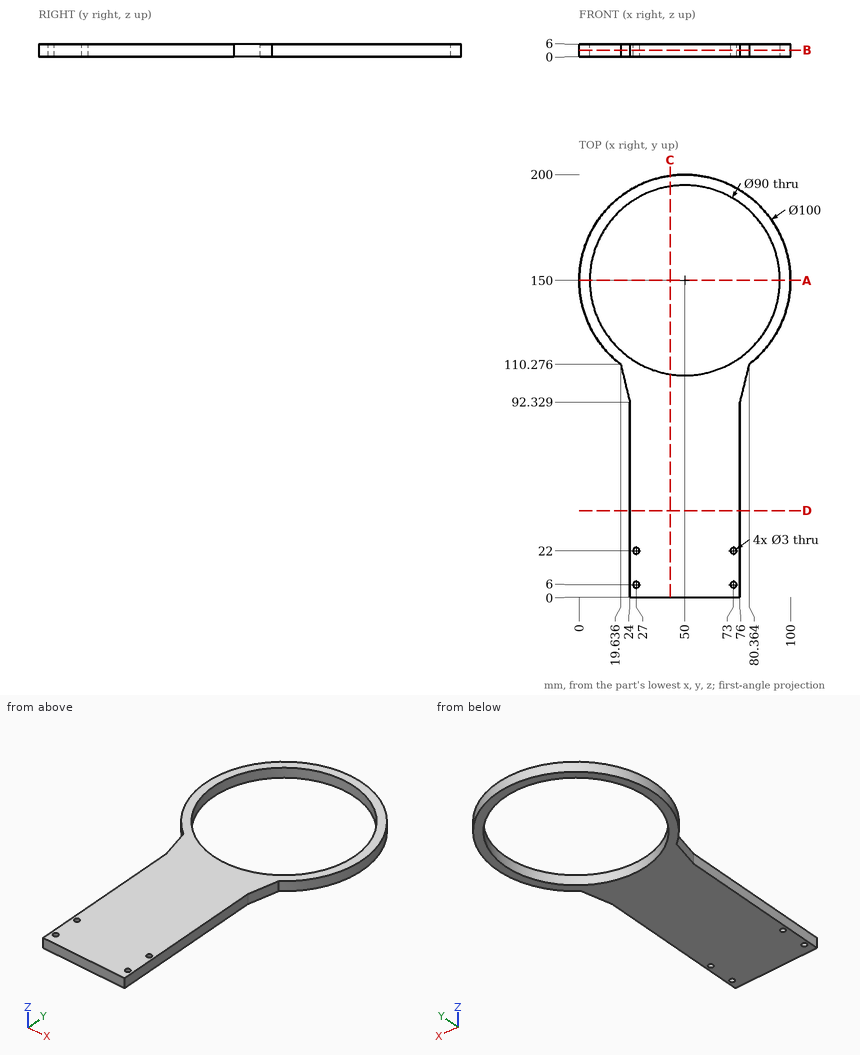
Study the drawing (mm; zero at the part's minimum x, y, z) and answer. Give positions to 0.01 mm unless a question says otherwise; leave off trailing zeros. Write each loop counter-clockwise with the first axis right and the second up, starting at its lowest first coordinate (ties: lowest second). Pieces come first, ordered by that corner, then holes. Notation, with made-up numbers: (13.5, 81) -> (57.5, 81) arc R9 cw to (57.5, 87) -> close; hole circle Ø3 at (-29.75, 11.25). An arc over 180 degrees is marked (long way). Answer as a JSON object with one key per item and string values. Group by question number.
1) Find section B-B (z = 3.15). Write down the section's boundary in (x, y).
2) Consider L1, parallel to X at y = 6, z = 3.1; L2, parallel to Y at x = 50, z = 4.85; L3, parallel to X at y = 148.5, z = 1.75 (1 decimal). Determine where each line is inside the solid, lowest interval first. Write a range as from..to.
3) Find section D-D (y = 41). Write down the section's boundary in (x, z), and give its area (3 significant figures).
4) Find section A-A (y = 150). Write down the section's boundary in (x, z).
5) Find section C-C (x = 43). Write down the section's boundary in (y, z).
6) This flat-tipped pin is pushed along its axis until it touches: P1, Ø1.8, axis at y = 41.5, z = 3.5, coming from the +X side. Where does it stop, or does it pass through?
Values follow:
{
 "1": {"outline": "(19.64, 110.28) -> (24, 92.33) -> (24, 0) -> (76, 0) -> (76, 92.33) -> (80.36, 110.28) arc R50 ccw (long way) to start; hole circle Ø90 at (50, 150); hole circle Ø3 at (27, 6); hole circle Ø3 at (27, 22); hole circle Ø3 at (73, 6); hole circle Ø3 at (73, 22)"},
 "2": {"L1": "x = 24..25.5, 28.5..71.5, 74.5..76", "L2": "y = 0..105, 195..200", "L3": "x = 0..5, 95..100"},
 "3": {"outline": "(24, 0) -> (76, 0) -> (76, 6) -> (24, 6) -> close", "area": "312 mm2"},
 "4": {"outline": "(0, 0) -> (5, 0) -> (5, 6) -> (0, 6) -> close; (95, 0) -> (100, 0) -> (100, 6) -> (95, 6) -> close"},
 "5": {"outline": "(0, 0) -> (105.55, 0) -> (105.55, 6) -> (0, 6) -> close; (194.45, 0) -> (199.51, 0) -> (199.51, 6) -> (194.45, 6) -> close"},
 "6": {"P1": "stops at x = 76"}
}
